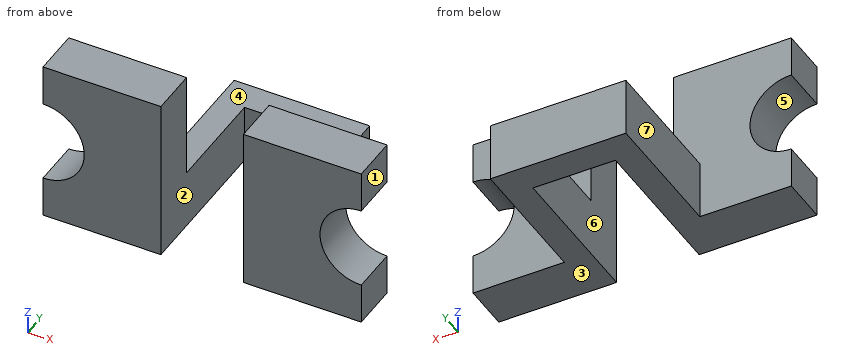
from build123d import *

# Parameters (mm, degrees)
EXTRUDE_1_DEPTH   = 8
EXTRUDE_1_2_DEPTH = 8
EXTRUDE_2_DEPTH   = 10


with BuildPart() as part:
    # Sketch 1 → Extrude 1 (new body)
    with BuildSketch(Plane(origin=(0, 0, 0), x_dir=(1, 0, 0), z_dir=(0, 1, 0))):
        with BuildLine():
            Line((27, 21), (27, 28))
            Line((27, 28), (7, 28))
            Line((7, 28), (7, 0))
            Line((7, 0), (27, 0))
            Line((27, 0), (27, 7))
            ThreePointArc((27, 7), (20, 14), (27, 21))
        make_face()
    extrude(amount=EXTRUDE_1_DEPTH)



with BuildPart() as body_2:
    # Sketch 1 → Extrude 1 2 (new body)
    with BuildSketch(Plane(origin=(0, 0, 0), x_dir=(1, 0, 0), z_dir=(0, 1, 0))):
        with BuildLine():
            Line((-27, 0), (-27, 7))
            ThreePointArc((-27, 7), (-20, 14), (-27, 21))
            Line((-27, 21), (-27, 28))
            Line((-27, 28), (-7, 28))
            Line((-7, 28), (-7, 0))
            Line((-7, 0), (-27, 0))
        make_face()
    extrude(amount=EXTRUDE_1_2_DEPTH)


with BuildPart() as part_1:
    add(part.part)

    add(body_2.part)  # Extrude 2 merges body 2
    # Sketch 2 → Extrude 2 (add)
    with BuildSketch(Plane(origin=(0, 0, -28), x_dir=(-1, 0, 0), z_dir=(0, 0, -1))):
        Polygon((-11.5, 31), (11.5, 31), (11.5, 8), (7, 8), (7, 26), (-7, 26), (-7, 8), (-11.5, 8), align=None)
    extrude(amount=-EXTRUDE_2_DEPTH)


solid = part_1.part
CAD build for the part. Positions are in the model's coordinates, mm. Face numbers are marked on the shaded views. A direction names the side the tool comes from. Coordinates: 2 decimals unless noted, no trailing zeros. Write each loop counter-clockwise with the first axis right and the second up, starting at its lowest first coordinate (ties: lowest second). Pieces come first, ordered by that corner, then holes. Notation, with made-up numbers: M -21.5,13.25 L -8.5,13.25 A25 ccw -8.5,37.25 Z; hole C 12,-26.5 d6. An arc over 180 degrees is marked long. Answer as a JSON object with one key per item and string values. Group by question number.
1) Saw through at C-C (x = -21.5). Write the cut outline in (y, z), plus the area to 3 significant figures.
2) Pin check, flat tips, straight feed: pin 1 Ø8 at (y, z) = (10, -11.5) entering from -X; pin 2 Ø11 at (x, z) = (0.5, -25) entering from -Y; pin 3 Ø1 at (x, z) = (9.5, -9) entering from +Y. Stop position of each tip, or through.
3) Saw through at D-D (x = -5). Write the cut outline in (y, z).
4) Tool access for the marked faces 4, 5, 6 and 7: list every direction of +Z, -Z, +X, -X, +Y, -Y with a clear straight run to the whole face (end or side of a thin tool).
5) Mould opens along X. For the marked faces 1, 2 and 3 say: +X half, -X half, draft (parallel to the pull), parting line (faces both ways), or undercut.
6) Saw through at A-A (y = 6.5). Write the cut outline in (x, z).
7) Saw through at B-B (z = -14). Write the cut outline in (x, y), plus the area to 3 significant figures.
8) Wall check: line 1 (X direction, y = 16.5, z = -24.75); line 2 (Y direction, x = 21.5, z = -9); line 3 (X direction, y = 6, z = -19.75). Give the ranges that are in metal, low to high. Write a range as from..to.
Values follow:
{
 "1": {"outline": "M 0,-28 L 8,-28 L 8,-18.33 L 0,-18.33 Z; M 0,-9.67 L 8,-9.67 L 8,0 L 0,0 Z", "area": "155 mm2"},
 "2": {"pin 1": "stops at x = -23.34", "pin 2": "stops at y = 26", "pin 3": "stops at y = 8"},
 "3": {"outline": "M 26,-28 L 31,-28 L 31,-18 L 26,-18 Z"},
 "4": {"face 4": "+Z, +X, -X, +Y", "face 5": "-X, +Y, -Y", "face 6": "+Z, -Z, -Y", "face 7": "+Z, -Z, -X, +Y"},
 "5": {"face 1": "+X half", "face 2": "undercut", "face 3": "draft"},
 "6": {"outline": "M -27,-28 L -7,-28 L -7,0 L -27,0 L -27,-7 A7 cw -27,-21 Z; M 7,-28 L 27,-28 L 27,-21 A7 cw 27,-7 L 27,0 L 7,0 Z"},
 "7": {"outline": "M -20,0 L -7,0 L -7,8 L -20,8 Z; M 7,0 L 20,0 L 20,8 L 7,8 Z", "area": "208 mm2"},
 "8": {"line 1": "x = -11.5..-7, 7..11.5", "line 2": "y = 0..8", "line 3": "x = -23.01..-7, 7..23.01"}
}
